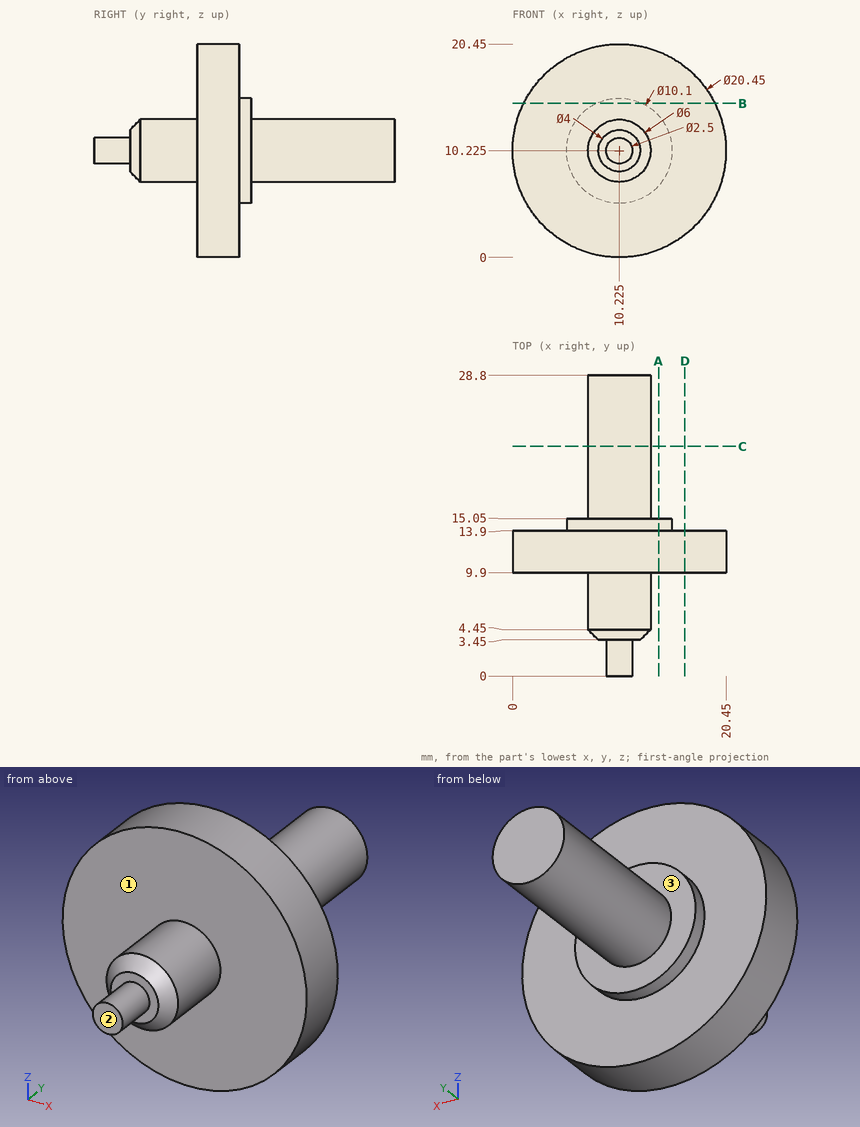
Part print with two shaded views. Sizes in mm from the minimum x, y, z corner. A direction names the side the tool comes from. Round coordinates to 2 decimals unless told otherwise and drop trailing zeros. Order: outer loops, then holes, each group sorted by start corner. A loop starts at its lowest first (then second) coordinate and runs counter-clockwise, first axis right, second up.
(1) Band-saw the part on B-B (z = 14.75). List the corners of the cut face in (x, y), then the cut area to 3 significant figures.
(2) 3-axis set-ups, long thin cutter, end or side, ignore diameter. For the marked faces 1, 2 and 3: which of +Z, -Z, +X, -X, +Y, -Y reach the whole face in a straight line?
(3) Band-saw the part on A-A (x = 14). List the corners of the cut face in (y, z), then the cut area to 3 significant figures.
(4) Band-saw the part on C-C (y = 22). List the corners of the cut face in (x, z) (3 decimals), then the cut area to 3 significant figures.
(5) Drill centre lines: line 1 (Y direction, x = 13.25, z = 4.5); line 2 (X direction, y = 16.25, z = 10); line 3 (X direction, y = 14.75, z = 10.5). Where is each one in solid material? Low to high.
(6) Pin check, flat tips, straight feed: pin 1 (3 mm diameter, centred on x = 13.5, y = 24, fed in from -Z); pin 2 (6 mm diameter, centred on x = 13, y = 22.5, fed in from -Z) (3 decimals); pin 3 (12 mm diameter, centred on x = 17.5, z = 16.5, fed in from +Y). Stop position of each tip, or through.
(7) Band-saw the part on D-D (x = 16.5). List the corners of the cut face in (y, z).
Verdict:
1. outline: (1.06, 9.9) - (19.39, 9.9) - (19.39, 13.9) - (12.47, 13.9) - (12.47, 15.05) - (7.98, 15.05) - (7.98, 13.9) - (1.06, 13.9) - close
1. area: 78.5 mm2
2. face 1: -Y
2. face 2: +Z, -Z, +X, -X, -Y
2. face 3: +Y
3. outline: (9.9, 0.72) - (13.9, 0.72) - (13.9, 6.87) - (15.05, 6.87) - (15.05, 13.58) - (13.9, 13.58) - (13.9, 19.73) - (9.9, 19.73) - close
3. area: 83.7 mm2
4. outline: circle Ø6 at (10.225, 10.225)
4. area: 28.3 mm2
5. line 1: y = 9.9 to 13.9
5. line 2: x = 7.23 to 13.22
5. line 3: x = 5.18 to 15.27
6. pin 1: stops at z = 7.81
6. pin 2: stops at z = 7.225
6. pin 3: stops at y = 15.05
7. outline: (9.9, 2.15) - (13.9, 2.15) - (13.9, 18.3) - (9.9, 18.3) - close
